Verification items for the finished model (mm, model axes). Coordinates: 2 decimals unless noted, no trailing zeros. Loops run counter-clockwise (first coordinate to the right, second up) from the corner with the lowest first, then second, coordinate; pieces in that order, holes last.
Q1. Sectioned sample at B-B (y = -30). Enter the section's corners in (x, z).
Q2. Sectioned sample at C-C (x = 229). Enter the section's corners in (y, z), then the cut area to 3 significant figures.
Q3. Sectioned sample at A-A (z = 2.15). Count the separate pieces of the cut face and the enclosed holes in it, then the cut area to 3 significant figures.
Q4. Mould release check, pull along Y, two halves, no side actions. Record for faces 1 (the face through (86, 1, 0)), 2 (the face through (232.91, -8.52, 2.46)): +Y half, -Y half, draft (parallel to the pull), parting line (faces both ways), or undercut.
Q5. Sectioned sample at D-D (x = 59). Enter the section's corners in (y, z).
Q6. Material ranges on probe 1 along Y at (x, z) = (202.42, 1.3); probe 2 along Y at (x, z) = (-77, 3.4); probe 3 along X at (y, z) = (30, 1.6), recorded low to high.
```python
from build123d import *

# Parameters (mm, degrees)
SKETCH1_W           = 350
SKETCH1_H           = 80
BOSS_EXTRUDE1_DEPTH = 5
SKETCH2_R           = 17.5
CUT_EXTRUDE1_DEPTH  = 60
SKETCH3_R           = 5.1
CUT_EXTRUDE2_DEPTH  = 10
SKETCH5_R           = 4.1
CUT_EXTRUDE3_DEPTH  = 267.071418984
SKETCH7_R           = 4.1
CUT_EXTRUDE5_DEPTH  = 267.071418984


with BuildPart() as part:
    # Sketch1 → Boss-Extrude1 (new body)
    with BuildSketch(Plane.XY):
        with Locations((88, 0)):
            Rectangle(SKETCH1_W, SKETCH1_H)
    extrude(amount=BOSS_EXTRUDE1_DEPTH)

    # Sketch2 → Cut-Extrude1 (cut)
    with BuildSketch(Plane(origin=(211.325798344, -35.262222233, -13.242737988), x_dir=(1, 0, 0), z_dir=(0, 0, 1))):
        with Locations((-211.325798344, 35.262222233)):
            Circle(SKETCH2_R)
    extrude(amount=CUT_EXTRUDE1_DEPTH, mode=Mode.SUBTRACT)

    # Sketch3 → Cut-Extrude2 (cut)
    with BuildSketch(Plane(origin=(20.819518943, -63.639721452, 0), x_dir=(1, 0, 0), z_dir=(0, 0, 1))):
        with Locations((-97.819518943, 93.639721452)):
            Circle(SKETCH3_R)
        with Locations(Location((38.180481057, 33.639721452, 0), (0, 0, 180))):
            Circle(SKETCH3_R)
        with Locations((38.180481057, 93.639721452)):
            Circle(SKETCH3_R)
        with Locations(Location((-97.819518943, 33.639721452, 0), (0, 0, 180))):
            Circle(SKETCH3_R)
    extrude(amount=CUT_EXTRUDE2_DEPTH, mode=Mode.SUBTRACT)

    # Sketch5 → Cut-Extrude3 (cut, through all)
    with BuildSketch(Plane.XY):
        with Locations((229, 9.75)):
            Circle(SKETCH5_R)
        with Locations((229, -9.75)):
            Circle(SKETCH5_R)
    extrude(amount=CUT_EXTRUDE3_DEPTH, mode=Mode.SUBTRACT)

    # Sketch7 → Cut-Extrude5 (cut, through all)
    with BuildSketch(Plane.XY):
        with Locations((202.42, 30)):
            Circle(SKETCH7_R)
        with Locations(Location((202.42, -30, 0), (0, 0, 180))):
            Circle(SKETCH7_R)
        with Locations((255.58, -30)):
            Circle(SKETCH7_R)
        with Locations(Location((255.58, 30, 0), (0, 0, 180))):
            Circle(SKETCH7_R)
    extrude(amount=CUT_EXTRUDE5_DEPTH, mode=Mode.SUBTRACT)


solid = part.part
```
Geometry check:
1. outline: (-87, 0) - (-82.1, 0) - (-82.1, 5) - (-87, 5) - close; (-71.9, 0) - (53.9, 0) - (53.9, 5) - (-71.9, 5) - close; (64.1, 0) - (198.32, 0) - (198.32, 5) - (64.1, 5) - close; (206.52, 0) - (251.48, 0) - (251.48, 5) - (206.52, 5) - close; (259.68, 0) - (263, 0) - (263, 5) - (259.68, 5) - close
2. outline: (-40, 0) - (-13.85, 0) - (-13.85, 5) - (-40, 5) - close; (-5.65, 0) - (5.65, 0) - (5.65, 5) - (-5.65, 5) - close; (13.85, 0) - (40, 0) - (40, 5) - (13.85, 5) - close
2. area: 318 mm2
3. separate pieces: 1
3. enclosed holes: 11
3. area: 26,400 mm2
4. face 1: draft
4. face 2: undercut
5. outline: (-40, 0) - (-35.1, 0) - (-35.1, 5) - (-40, 5) - close; (-24.9, 0) - (24.9, 0) - (24.9, 5) - (-24.9, 5) - close; (35.1, 0) - (40, 0) - (40, 5) - (35.1, 5) - close
6. probe 1: y = -40 to -34.1, -25.9 to 25.9, 34.1 to 40
6. probe 2: y = -40 to -35.1, -24.9 to 24.9, 35.1 to 40
6. probe 3: x = -87 to -82.1, -71.9 to 53.9, 64.1 to 198.32, 206.52 to 251.48, 259.68 to 263
